Verification items for the finished model (mm, model axes). A direction names the side the tool comes from. Round coordinates to 2 decimals unless told otherwise and drop trailing zeros. Order: outer loops, then holes, each group sorted by start corner. A loop starts at its lowest first (then second) coordinate and runs counter-clockwise, first axis right, second up. Notation, with made-up numbers: (22, -16.5) -> (34, -16.5) arc R20 ccw to (34, 1.5) -> close; hole circle Ø9 at (50.5, -36.75). An arc over 180 degrees is marked (long way). Return JSON: item names as keys, results as strings. Group by question number.
Item 1: Sectioned sample at C-C on y = 7. Record the cut outline in (x, z) (3 decimals).
Item 2: Sectioned sample at B-B on x = 0.5. Record the cut outline in (y, z) (3 decimals), plus the area to 3 significant figures.
Item 3: Depth check by flat-ended pin: pin 1 Ø4.5 at (x, z) = (0, -28.5) entering from -Y; pin 2 Ø1.6 at (x, z) = (0, -28) entering from +Y; pin 3 Ø6 at (x, z) = (-7, -16.5) entering from -Y; pin 4 Ø2 at (x, y) = (1, 13) entering from -Z (3 decimals). Enter the tip coordinate at first touch or a pass-through.
Item 4: Sectioned sample at D-D on x = -6. Record the cut outline in (y, z) (3 decimals), plus the area to 3 significant figures.
Item 5: Access from +Z, -Z, +X, -X, +Y, -Y to the whole of each face (thin tool, end or side, straight path). Record for faces 1 (the flat face through (0, 8.87, 28)), 2 (the flat face through (-4.375, 5, 28)), 3 (the flat face through (0, 2, -28)), 4 (the flat face through (0, 2, 28)).
Item 6: Scan lines: probe 1 along Z at (x, y) = (-11, 9) (3 decimals); probe 2 along X at (y, z) = (5.75, 26.5) (3 decimals); probe 3 along Y at (x, z) = (-1, -27.5). Record each from-to range of solid material in increasing order. Write a range as from..to.
Item 7: Sectioned sample at A-A on y = 10.25. Record the cut outline in (x, z) (3 decimals), plus the area to 3 significant figures.
```python
from build123d import *

# Parameters (mm, degrees)
SKETCH1_W           = 32.3
SKETCH1_H           = 51.25
BOSS_EXTRUDE2_DEPTH = 16.6
SKETCH2_W           = 8.75
SKETCH2_H           = 6.87
BOSS_EXTRUDE3_DEPTH = 5.5
SKETCH3_W           = 8.75
SKETCH3_H           = 6.929487278
BOSS_EXTRUDE4_DEPTH = 5.5
FILLET1_R           = 0.8


with BuildPart() as part:
    # Sketch1 → Boss-Extrude2 (new body)
    with BuildSketch(Plane(origin=(0, 0, 0), x_dir=(1, 0, 0), z_dir=(0, 1, 0))):
        Rectangle(SKETCH1_W, SKETCH1_H)
    extrude(amount=BOSS_EXTRUDE2_DEPTH)

    # Sketch2 → Boss-Extrude3 (add)
    with BuildSketch(Plane.XY.offset(25.625)):
        with Locations((0, 5.435)):
            Rectangle(SKETCH2_W, SKETCH2_H)
    extrude(amount=BOSS_EXTRUDE3_DEPTH)

    # Sketch3 → Boss-Extrude4 (add)
    with BuildSketch(Plane(origin=(0, 0, -25.625), x_dir=(-1, 0, 0), z_dir=(0, 0, -1))):
        with Locations((0, 5.464743639)):
            Rectangle(SKETCH3_W, SKETCH3_H)
    extrude(amount=BOSS_EXTRUDE4_DEPTH)

    # Fillet1
    fillet1_edges = [part.edges().sort_by_distance(p)[0] for p in [
        (-4.375, 5.435, 31.125),
        (4.375, 5.435, 31.125),
        (4.375, 5.464743639, -31.125),
        (-4.375, 5.464743639, -31.125),
        (-16.15, 8.3, -25.625),
        (16.15, 8.3, -25.625),
        (16.15, 8.3, 25.625),
        (-16.15, 8.3, 25.625),
    ]]
    fillet(fillet1_edges, radius=FILLET1_R)


solid = part.part
```
Recorded:
{
 "1": {"outline": "(-16.15, -24.825) arc R0.8 ccw to (-15.35, -25.625) -> (-4.375, -25.625) -> (-4.375, -30.325) arc R0.8 ccw to (-3.575, -31.125) -> (3.575, -31.125) arc R0.8 ccw to (4.375, -30.325) -> (4.375, -25.625) -> (15.35, -25.625) arc R0.8 ccw to (16.15, -24.825) -> (16.15, 24.825) arc R0.8 ccw to (15.35, 25.625) -> (4.375, 25.625) -> (4.375, 30.325) arc R0.8 ccw to (3.575, 31.125) -> (-3.575, 31.125) arc R0.8 ccw to (-4.375, 30.325) -> (-4.375, 25.625) -> (-15.35, 25.625) arc R0.8 ccw to (-16.15, 24.825) -> close"},
 "2": {"outline": "(0, -25.625) -> (2, -25.625) -> (2, -31.125) -> (8.929, -31.125) -> (8.929, -25.625) -> (16.6, -25.625) -> (16.6, 25.625) -> (8.87, 25.625) -> (8.87, 31.125) -> (2, 31.125) -> (2, 25.625) -> (0, 25.625) -> close", "area": "927 mm²"},
 "3": {"pin 1": "y = 2", "pin 2": "y = 8.93", "pin 3": "y = 0", "pin 4": "z = -25.625"},
 "4": {"outline": "(0, -25.625) -> (16.6, -25.625) -> (16.6, 25.625) -> (0, 25.625) -> close", "area": "851 mm²"},
 "5": {"face 1": "+Z, +X, -X, +Y", "face 2": "+Z, -X, +Y, -Y", "face 3": "-Z, +X, -X, -Y", "face 4": "+Z, +X, -X, -Y"},
 "6": {"probe 1": "-25.625..25.625", "probe 2": "-4.375..4.375", "probe 3": "2..8.93"},
 "7": {"outline": "(-16.15, -24.825) arc R0.8 ccw to (-15.35, -25.625) -> (15.35, -25.625) arc R0.8 ccw to (16.15, -24.825) -> (16.15, 24.825) arc R0.8 ccw to (15.35, 25.625) -> (-15.35, 25.625) arc R0.8 ccw to (-16.15, 24.825) -> close", "area": "1,650 mm²"}
}
